Can you work these out from the model? Positions are in its coordinate system, mm. A direction names the side the tool comes from. Coordinates: 2 decimals unless noted, no trailing zeros. Loops run counter-clockwise (first coordinate to the right, second up) from the corner with the lowest first, then second, coordinate; pieces in that order, holes last. Notation, with made-up numbers: (21.25, 88.5) -> (72.25, 88.5) arc R12 ccw to (72.25, 106.5) -> close; hole circle Ø2 at (46.25, 45.5). An arc over 180 degrees is marked (long way). Put each result on its own line as item: value. Start each with the question number.
Item 1: For faces 1 (the cylindrical face through (-1.721, -11.917, 180.485)), 2 (the flat face through (25.4, 0, 150)), 3 (the cylindrical face through (-1.86, 11.917, 245.734)), 4 (the flat face through (-23.812, 0, 150)), which set-ups out of +Z, -Z, +X, -X, +Y, -Y let a thin tool reach every point of the face, with its end or its side?
Item 2: Please list where these lines run through material, in increasing order: L1, parallel to X at y = 8.25, z = 51; L2, parallel to Y at x = 22, z = 211; L3, parallel to Z at x = 0, y = 11.7. Write a range as from..to.
Item 3: If we section it at A-A on y = -8.5: Please give me the cut outline in (x, z), plus the area to 3 significant figures.
Item 4: If we section it at D-D on z = 106: Please give me the cut outline in (x, y) (1 decimal), plus the area to 3 significant figures.
Item 5: Will these pins go through, and if not, where does the flat tip stop? P1, Ø4, axis at x = 0, z = 116.57, coming from the +Y side; P2, Ø20.5, axis at x = 0, z = 188.23, coming from the +Y side.
Item 6: We'd pull the mould along X, two halves only. Please class faces 5 (the flat face through (-25.4, 0, 150)), 6 (the flat face through (0, 11.112, 150)), 7 (the flat face through (0, -12, 0)): pulls with the +X half, pulls with the -X half, needs draft (parallel to the pull), parting line crosses it, or undercut.
Item 7: If we section it at C-C on x = -19: Please give me the cut outline in (y, z), plus the area to 3 significant figures.
Item 8: If we section it at B-B on z = 44.9: Please give me the cut outline in (x, y) (1 decimal).
```python
from build123d import *

# Parameters (mm, degrees)
SKETCH1_W                      = 47.625
SKETCH1_H                      = 22.225
BOSS_EXTRUDE1_DEPTH            = 304.8
CUT_EXTRUDE1_REACH             = 27.4
SKETCH2_R                      = 14.2875
CUT_EXTRUDE1_DIRECTION_2_DEPTH = 1
CUT_EXTRUDE2_REACH             = 27.4
SKETCH3_R                      = 12.7
CUT_EXTRUDE2_DIRECTION_2_DEPTH = 1
CUT_EXTRUDE3_REACH             = 27.4
SKETCH4_R                      = 3.3782
CUT_EXTRUDE3_DIRECTION_2_DEPTH = 1
CUT_EXTRUDE4_REACH             = 27.4
SKETCH5_R                      = 7.9375
CUT_EXTRUDE4_DIRECTION_2_DEPTH = 1


with BuildPart() as part:
    # Sketch1 → Boss-Extrude1 (new body)
    with BuildSketch(Plane.XY):
        with BuildLine():
            Line((-23.8125, -12.7), (23.8125, -12.7))
            ThreePointArc((23.8125, -12.7), (24.935032015, -12.235032015), (25.4, -11.1125))
            Line((25.4, -11.1125), (25.4, 11.1125))
            ThreePointArc((25.4, 11.1125), (24.935032015, 12.235032015), (23.8125, 12.7))
            Line((23.8125, 12.7), (-23.8125, 12.7))
            ThreePointArc((-23.8125, 12.7), (-24.935032015, 12.235032015), (-25.4, 11.1125))
            Line((-25.4, 11.1125), (-25.4, -11.1125))
            ThreePointArc((-25.4, -11.1125), (-24.935032015, -12.235032015), (-23.8125, -12.7))
        make_face()
        Rectangle(SKETCH1_W, SKETCH1_H, mode=Mode.SUBTRACT)
    extrude(amount=BOSS_EXTRUDE1_DEPTH)

    # Sketch2 → Cut-Extrude1 (cut, up to next)
    with BuildSketch(Plane(origin=(0, 12.7, 0), x_dir=(1, 0, 0), z_dir=(0, 1, 0)), mode=Mode.PRIVATE) as cut_extrude1_sk1:
        with Locations((0, -259.900000011)):
            Circle(SKETCH2_R)
    cut_extrude1_tool1 = extrude(cut_extrude1_sk1.sketch, amount=-CUT_EXTRUDE1_REACH, mode=Mode.PRIVATE) & part.part
    add(cut_extrude1_tool1.solids().sort_by_distance((0, 12.7, 259.9))[0], mode=Mode.SUBTRACT)
    # Sketch2 → Cut-Extrude1 (cut, up to next)
    with BuildSketch(Plane(origin=(0, 12.7, 0), x_dir=(1, 0, 0), z_dir=(0, 1, 0)), mode=Mode.PRIVATE) as cut_extrude1_sk2:
        with Locations((0, -44.899999989)):
            Circle(SKETCH2_R)
    cut_extrude1_tool2 = extrude(cut_extrude1_sk2.sketch, amount=-CUT_EXTRUDE1_REACH, mode=Mode.PRIVATE) & part.part
    add(cut_extrude1_tool2.solids().sort_by_distance((0, 12.7, 44.9))[0], mode=Mode.SUBTRACT)

    # Sketch2 → Cut-Extrude1 direction 2 (cut)
    with BuildSketch(Plane(origin=(0, 12.7, 0), x_dir=(1, 0, 0), z_dir=(0, 1, 0))):
        with Locations((0, -259.900000011)):
            Circle(SKETCH2_R)
        with Locations((0, -44.899999989)):
            Circle(SKETCH2_R)
    extrude(amount=CUT_EXTRUDE1_DIRECTION_2_DEPTH, mode=Mode.SUBTRACT)

    # Sketch3 → Cut-Extrude2 (cut, up to next)
    with BuildSketch(Plane.XZ.offset(12.7), mode=Mode.PRIVATE) as cut_extrude2_sk1:
        with Locations((0, 44.899999989)):
            Circle(SKETCH3_R)
    cut_extrude2_tool1 = extrude(cut_extrude2_sk1.sketch, amount=-CUT_EXTRUDE2_REACH, mode=Mode.PRIVATE) & part.part
    add(cut_extrude2_tool1.solids().sort_by_distance((0, -12.7, 44.9))[0], mode=Mode.SUBTRACT)
    # Sketch3 → Cut-Extrude2 (cut, up to next)
    with BuildSketch(Plane.XZ.offset(12.7), mode=Mode.PRIVATE) as cut_extrude2_sk2:
        with Locations((0, 259.900000011)):
            Circle(SKETCH3_R)
    cut_extrude2_tool2 = extrude(cut_extrude2_sk2.sketch, amount=-CUT_EXTRUDE2_REACH, mode=Mode.PRIVATE) & part.part
    add(cut_extrude2_tool2.solids().sort_by_distance((0, -12.7, 259.9))[0], mode=Mode.SUBTRACT)

    # Sketch3 → Cut-Extrude2 direction 2 (cut)
    with BuildSketch(Plane.XZ.offset(12.7)):
        with Locations((0, 44.899999989)):
            Circle(SKETCH3_R)
        with Locations((0, 259.900000011)):
            Circle(SKETCH3_R)
    extrude(amount=CUT_EXTRUDE2_DIRECTION_2_DEPTH, mode=Mode.SUBTRACT)

    # Sketch4 → Cut-Extrude3 (cut, up to next)
    with BuildSketch(Plane(origin=(0, 12.7, 0), x_dir=(1, 0, 0), z_dir=(0, 1, 0)), mode=Mode.PRIVATE) as cut_extrude3_sk1:
        with Locations((0, -188.233332829)):
            Circle(SKETCH4_R)
    cut_extrude3_tool1 = extrude(cut_extrude3_sk1.sketch, amount=-CUT_EXTRUDE3_REACH, mode=Mode.PRIVATE) & part.part
    add(cut_extrude3_tool1.solids().sort_by_distance((0, 12.7, 188.233333))[0], mode=Mode.SUBTRACT)
    # Sketch4 → Cut-Extrude3 (cut, up to next)
    with BuildSketch(Plane(origin=(0, 12.7, 0), x_dir=(1, 0, 0), z_dir=(0, 1, 0)), mode=Mode.PRIVATE) as cut_extrude3_sk2:
        with Locations((0, -116.566667171)):
            Circle(SKETCH4_R)
    cut_extrude3_tool2 = extrude(cut_extrude3_sk2.sketch, amount=-CUT_EXTRUDE3_REACH, mode=Mode.PRIVATE) & part.part
    add(cut_extrude3_tool2.solids().sort_by_distance((0, 12.7, 116.566667))[0], mode=Mode.SUBTRACT)

    # Sketch4 → Cut-Extrude3 direction 2 (cut)
    with BuildSketch(Plane(origin=(0, 12.7, 0), x_dir=(1, 0, 0), z_dir=(0, 1, 0))):
        with Locations((0, -188.233332829)):
            Circle(SKETCH4_R)
        with Locations((0, -116.566667171)):
            Circle(SKETCH4_R)
    extrude(amount=CUT_EXTRUDE3_DIRECTION_2_DEPTH, mode=Mode.SUBTRACT)

    # Sketch5 → Cut-Extrude4 (cut, up to next)
    with BuildSketch(Plane.XZ.offset(12.7), mode=Mode.PRIVATE) as cut_extrude4_sk1:
        with Locations((0, 116.566667171)):
            Circle(SKETCH5_R)
    cut_extrude4_tool1 = extrude(cut_extrude4_sk1.sketch, amount=-CUT_EXTRUDE4_REACH, mode=Mode.PRIVATE) & part.part
    add(cut_extrude4_tool1.solids().sort_by_distance((0, -12.7, 116.566667))[0], mode=Mode.SUBTRACT)
    # Sketch5 → Cut-Extrude4 (cut, up to next)
    with BuildSketch(Plane.XZ.offset(12.7), mode=Mode.PRIVATE) as cut_extrude4_sk2:
        with Locations((0, 188.233332829)):
            Circle(SKETCH5_R)
    cut_extrude4_tool2 = extrude(cut_extrude4_sk2.sketch, amount=-CUT_EXTRUDE4_REACH, mode=Mode.PRIVATE) & part.part
    add(cut_extrude4_tool2.solids().sort_by_distance((0, -12.7, 188.233333))[0], mode=Mode.SUBTRACT)

    # Sketch5 → Cut-Extrude4 direction 2 (cut)
    with BuildSketch(Plane.XZ.offset(12.7)):
        with Locations((0, 116.566667171)):
            Circle(SKETCH5_R)
        with Locations((0, 188.233332829)):
            Circle(SKETCH5_R)
    extrude(amount=CUT_EXTRUDE4_DIRECTION_2_DEPTH, mode=Mode.SUBTRACT)


solid = part.part
```
Solutions:
1. face 1: -Y
1. face 2: +Z, -Z, +X, +Y, -Y
1. face 3: +Y
1. face 4: +Z, -Z
2. L1: -25.4..-23.81, 23.81..25.4
2. L2: -12.7..-11.11, 11.11..12.7
2. L3: 0..30.61, 59.19..113.19, 119.94..184.86, 191.61..245.61, 274.19..304.8
3. outline: (-25.4, 0) -> (-23.81, 0) -> (-23.81, 304.8) -> (-25.4, 304.8) -> close; (23.81, 0) -> (25.4, 0) -> (25.4, 304.8) -> (23.81, 304.8) -> close
3. area: 968 mm^2
4. outline: (-25.4, -11.1) arc R1.6 ccw to (-23.8, -12.7) -> (23.8, -12.7) arc R1.6 ccw to (25.4, -11.1) -> (25.4, 11.1) arc R1.6 ccw to (23.8, 12.7) -> (-23.8, 12.7) arc R1.6 ccw to (-25.4, 11.1) -> close; hole (-23.8, -11.1) -> (23.8, -11.1) -> (23.8, 11.1) -> (-23.8, 11.1) -> close
4. area: 230 mm^2
5. P1: through
5. P2: y = 12.7
6. face 5: pulls with the -X half
6. face 6: undercut
6. face 7: needs draft
7. outline: (-12.7, 0) -> (-11.11, 0) -> (-11.11, 304.8) -> (-12.7, 304.8) -> close; (11.11, 0) -> (12.7, 0) -> (12.7, 304.8) -> (11.11, 304.8) -> close
7. area: 968 mm^2
8. outline: (-25.4, -11.1) arc R1.6 ccw to (-23.8, -12.7) -> (-12.7, -12.7) -> (-12.7, -11.1) -> (-23.8, -11.1) -> (-23.8, 11.1) -> (-14.3, 11.1) -> (-14.3, 12.7) -> (-23.8, 12.7) arc R1.6 ccw to (-25.4, 11.1) -> close; (12.7, -12.7) -> (23.8, -12.7) arc R1.6 ccw to (25.4, -11.1) -> (25.4, 11.1) arc R1.6 ccw to (23.8, 12.7) -> (14.3, 12.7) -> (14.3, 11.1) -> (23.8, 11.1) -> (23.8, -11.1) -> (12.7, -11.1) -> close
